Design review of the part built by this model. Coordinates are the model's own, in mm. Round coordinates to 2 decimals unless told otherwise and drop trailing zeros. Order: outer loops, then holes, each group sorted by start corner. A loop starts at its lowest first (then second) coordinate and runs counter-clockwise, first axis right, second up.
from build123d import *

# Parameters (mm, degrees)
ESQUISSE1_W             = 639
ESQUISSE1_H             = 48
BOSS_EXTRU_1_DEPTH      = 24
ENL_V_MAT_EXTRU_1_DEPTH = 322.297759096
ESQUISSE3_R             = 4.5
ENL_V_MAT_EXTRU_2_DEPTH = 322.297759096
ESQUISSE5_R             = 5
ENL_V_MAT_EXTRU_4_DEPTH = 324.975693533
ENL_V_MAT_EXTRU_5_DEPTH = 322.297759096


with BuildPart() as part:
    # Esquisse1 → Boss.-Extru.1 (new body)
    with BuildSketch(Plane.XY):
        Rectangle(ESQUISSE1_W, ESQUISSE1_H)
    extrude(amount=BOSS_EXTRU_1_DEPTH)

    # Esquisse2 → Enlèv. mat.-Extru.1 (cut, through all)
    with BuildSketch(Plane.XY.offset(24)):
        Polygon((-319.5, 24), (-271.5, -24), (-319.5, -24), align=None)
        Polygon((319.5, 24), (271.5, -24), (319.5, -24), align=None)
    extrude(amount=-ENL_V_MAT_EXTRU_1_DEPTH, mode=Mode.SUBTRACT)

    # Esquisse3 → Enlèv. mat.-Extru.2 (cut, through all)
    with BuildSketch(Plane.XY.offset(24)):
        with Locations((-200, 0)):
            Circle(ESQUISSE3_R)
        with Locations((200, 0)):
            Circle(ESQUISSE3_R)
    extrude(amount=-ENL_V_MAT_EXTRU_2_DEPTH, mode=Mode.SUBTRACT)

    # Esquisse5 → Enlèv. mat.-Extru.4 (cut, through all)
    with BuildSketch(Plane(origin=(0, 24, 0), x_dir=(1, 0, 0), z_dir=(0, 1, 0))):
        with Locations(Location((-150, -10, 0), (0, 0, 180))):
            Circle(ESQUISSE5_R)
        with Locations(Location((150, -10, 0), (0, 0, 180))):
            Circle(ESQUISSE5_R)
    extrude(amount=-ENL_V_MAT_EXTRU_4_DEPTH, mode=Mode.SUBTRACT)

    # Esquisse6 → Enlèv. mat.-Extru.5 (cut, through all)
    with BuildSketch(Plane(origin=(0, 0, 0), x_dir=(-1, 0, 0), z_dir=(0, 0, -1))):
        Polygon((-270, -25.5), (-270, 24), (-319.5, 24), align=None)
        Polygon((270, -25.5), (319.5, 24), (270, 24), align=None)
    extrude(amount=-ENL_V_MAT_EXTRU_5_DEPTH, mode=Mode.SUBTRACT)


solid = part.part
1) Take a section at A-A on x = 200. Give the boundary of the cut face in (y, z).
Results:
outline: (-24, 0) - (-4.5, 0) - (-4.5, 24) - (-24, 24) - close; (4.5, 0) - (24, 0) - (24, 24) - (4.5, 24) - close
2) Clearance check with flat-ended pins moving along their axes: P1, Ø14.5, axis at x = -200, y = 0, coming from the +Z side; P2, Ø8, axis at x = 150, z = 10, coming from the +Y side. State where each tip first meets the part, or that it passes through.
Results:
P1: stops at z = 24
P2: passes through
3) The part is to be moulded in two halves that separate along Y. For faces 1 (the face through (-4, 24, 12)), 2 (the face through (204.16, -1.72, 12.17)), 3 (the face through (-270, 0, 12)), say which applies: released by +Y, released by -Y, zero draft, split by the parting line, or undercut.
Results:
face 1: released by +Y
face 2: undercut
face 3: zero draft
4) To check wall thickness, follow line 1 along Y through (x, z) = (-200, 6.75); line 2 along Z through (x, y) = (-150, 1.5); line 3 along X through (y, z) = (19.5, 11.75). State the ranges of each line that lie inside material, in increasing order.
Results:
line 1: y = -24 to -4.5, 4.5 to 24
line 2: z = 0 to 5, 15 to 24
line 3: x = -270 to -154.68, -145.32 to 145.32, 154.68 to 270
